```python
from build123d import *

# Parameters (mm, degrees)
BOSS_EXTRUDE1_DEPTH = 3


with BuildPart() as part:
    # Sketch2 → Boss-Extrude1 (new body)
    with BuildSketch(Plane(origin=(0, 0, 0), x_dir=(1, 0, 0), z_dir=(0, 1, 0))):
        with BuildLine():
            Line((26.055569119, 8.188046441), (26.055569119, -15.511162218))
            Line((26.055569119, -15.511162218), (-26.055569119, -15.511162218))
            Line((-26.055569119, -15.511162218), (-26.055569119, 8.188046441))
            ThreePointArc((-26.055569119, 8.188046441), (-21.514872246, 4.669726518), (-15.870079226, 5.73406431))
            ThreePointArc((-15.870079226, 5.73406431), (-10.616247764, 4.133629141), (-7, 0))
            ThreePointArc((-7, 0), (0, -7), (7, 0))
            ThreePointArc((7, 0), (10.616247764, 4.133629141), (15.870079226, 5.73406431))
            ThreePointArc((15.870079226, 5.73406431), (21.514872246, 4.669726518), (26.055569119, 8.188046441))
        make_face()
    extrude(amount=BOSS_EXTRUDE1_DEPTH)


solid = part.part
```
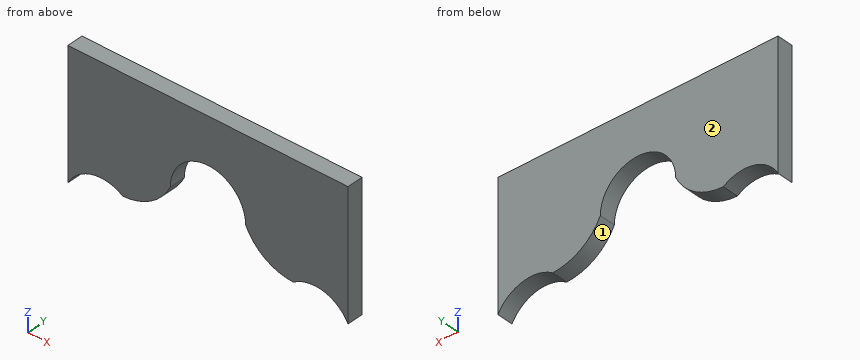
Input: part model. Units: mm. Frame: model coordinates. Face numbers are marked on the shaded views. Coordinates: 2 decimals unless noted, no trailing zeros. Loops run counter-clockwise (first coordinate to the right, second up) from the corner with the lowest first, then second, coordinate; pieces in that order, holes last. Notation, with made-up numbers: M 59.5,36 L 71.5,36 A20 cw 71.5,64 Z; hole C 69.5,21 d4. An arc over 180 degrees is marked long. Use a Markdown table: item, result. Add a question column.
1) Section B-B, the plane y = 2.1. Return the cut outline in (x, z) (3 decimals), plus the area to 3 significant figures.
2) Pin query (flat end, axial travel): P1, Ø8, axis at x = 3.5, z = 1.5, coming from the -Y side. Return the tip coordinate at first contact, or that it passes through.
3) Section A-A, the plane z = 4. Return the cut outline in (x, y).
4) Section C-C, the plane x = 0. Return the cut outline in (y, z).
5) Draft query along X for the marked faces 1 and 2. Return one class per face: +X half, -X half, draft (parallel to the pull), parting line (faces both ways), or undercut.
6) Line query: L1, parallel to X at y = 2.7, z = -6.25; L2, parallel to X at y = 1.5, z = -4.25; L3, parallel to Z at x = -14.5, y = 0.1. Output: solid intervals per line, ascending. Write a range as from..to.
Answer below:
| question | item | result |
|---|---|---|
| 1 | outline | M -26.056,-8.188 A7 cw -15.87,-5.734 A10 ccw -7,0 A7 cw 7,0 A10 ccw 15.87,-5.734 A7 cw 26.056,-8.188 L 26.056,15.511 L -26.056,15.511 Z |
| 1 | area | 911 mm2 |
| 2 | P1 | y = 0 |
| 3 | outline | M -26.06,0 L -5.74,0 L -5.74,3 L -26.06,3 Z; M 5.74,0 L 26.06,0 L 26.06,3 L 5.74,3 Z |
| 4 | outline | M 0,7 L 3,7 L 3,15.51 L 0,15.51 Z |
| 5 | face 1 | undercut |
| 5 | face 2 | draft |
| 6 | L1 | -26.06..-24.53, 24.53..26.06 |
| 6 | L2 | -26.06..-10.8, 10.8..26.06 |
| 6 | L3 | -5.62..15.51 |
